Autodesk Inventor part; units mm, degrees
ref_plane "YZ Plane" through (0, 0, 0) normal (1, 0, 0) x (0, 1, 0)
ref_plane "XZ Plane" through (0, 0, 0) normal (0, 1, 0) x (-1, 0, 0)
ref_plane "XY Plane" through (0, 0, 0) normal (0, 0, 1) x (1, 0, 0)
sketch "Sketch1" plane through (0, 0, 0) normal (0, 0, 1) x (1, 0, 0)
  line L0 (18.1, 0) -> (18.1, 27)
  line L1 (18.1, 27) -> (-0.25, 27)
  line L2 (0, 0) -> (18.1, 0)
  circle A0 centre (13.6, 6.8375) radius 2.5
  circle A1 centre (13.6, 20.1625) radius 2.5
  line L3 (-104.55, 27) -> (-122.9, 27)
  line L4 (-122.9, 0) -> (-122.9, 27)
  line L5 (-104.55, 0) -> (-122.9, 0)
  circle A2 centre (-118.4, 6.8375) radius 2.5
  circle A3 centre (-118.4, 20.1625) radius 2.5
  line L6 (-104.55, 27) -> (-0.25, 27)
  line L7 (-104.55, 0) -> (0, 0)
extrude "Extrusion1" add sketch "Sketch1" along normal blind 10
hole "Hole1" at (13.6, 20.1625, 10) direction (0, 0, -1) diameter 8 depth 2
hole "Hole2" at (13.6, 6.8375, 10) direction (0, 0, -1) diameter 8 depth 2
hole "Hole3" at (-118.4, 20.1625, 10) direction (0, 0, -1) diameter 8 depth 2
hole "Hole4" at (-118.4, 6.8375, 10) direction (0, 0, -1) diameter 8 depth 2
chamfer "Chamfer1" [suppressed]
sketch "Sketch2" plane through (0, 0, 0) normal (0, 1, 0) x (-1, 0, 0)
  line L0 (-18.1, 0) -> (104.6, 0) construction
  circle A0 centre (6.05, 0) radius 5.75
  circle A1 centre (29.25, 0) radius 5.75
  circle A2 centre (52.45, 0) radius 5.75
  circle A3 centre (29.25, 0) radius 5.75
  circle A4 centre (75.65, 0) radius 5.75
  circle A5 centre (98.85, 0) radius 5.75
  line L1 (-18.1, 0) -> (0, 0) construction
  line L2 (122.9, 0) -> (122.9, 10)
  line L3 (122.9, 0) -> (122.9, 10)
  line L4 (-18.1, 0) -> (-18.1, 10)
  line L5 (-18.1, 0) -> (-18.1, 10)
  dimension "d49" = 11.5
  dimension "d50" = 23.2
  dimension "d51" = 23.2
  dimension "d52" = 23.2
  dimension "d54" = 23.2
  dimension "d55" = 23.2
extrude "Extrusion2" cut sketch "Sketch2" along normal through all
sketch "Sketch3" plane through (0, 0, 0) normal (0, 0, 1) x (1, 0, 0)
  line L0 (-69.9, 0) -> (-69.9, 27)
  line L1 (-58.2, 27) -> (-69.9, 27)
  line L2 (-58.2, 27) -> (-58.2, 0)
  line L3 (-69.9, 0) -> (-58.2, 0)
  line L4 (-35, 27) -> (-35, 0)
  line L5 (-46.7, 0) -> (-35, 0)
  line L6 (-46.7, 0) -> (-46.7, 27)
  line L7 (-35, 27) -> (-46.7, 27)
  circle A0 centre (-64.05, 13.5) radius 2.6
  circle A1 centre (-40.85, 13.5) radius 2.6
  line L8 (-69.9, 0) -> (-69.9, 27)
  line L9 (-69.9, 13.5) -> (-35, 13.5) construction
  line L10 (-64.05, 0) -> (-64.05, 27) construction
  line L11 (-122.9, 0) -> (18.1, 0)
  line L12 (-40.85, 0) -> (-40.85, 27) construction
  point P0 (0, 0)
  point P1 (-40.85, 13.5)
  dimension "d66" = 5.2
extrude "Extrusion3" cut sketch "Sketch3" along normal through all contours A0 | A1
hole "Hole5" at (-40.85, 13.5, 10) direction (0, 0, -1) diameter 9.5 depth 3
hole "Hole6" at (-64.05, 13.5, 10) direction (0, 0, -1) diameter 9.5 depth 3
equation "\"d51\" = d50"
equation "\"d52\" = d50"
equation "\"d54\" = d50"
properties part number "cylinder-holder-1" material "Nylon 6/6"
The model under review builds one solid part; all positions refer to its coordinate system, in mm. A direction names the side the tool comes from. Round coordinates to 2 decimals unless told otherwise and drop trailing zeros. Order: outer loops, then holes, each group sorted by start corner. A loop starts at its lowest first (then second) coordinate and runs counter-clockwise, first axis right, second up. Notation, with made-up numbers: (-28, 5.25) - (-5, 5.25) arc R20 ccw to (-5, 10.25) - close; hole circle Ø5 at (-34, 12). An arc over 180 degrees is marked (long way). Use one line per item in the form item = value.
Q1. Add section B-B on y = 13.5. Give the number of separate pieces and of enclosed holes in the cut face, then the cut area to 3 significant figures.
Response values:
separate_pieces = 3
enclosed_holes = 0
area = 1,020 mm^2
Q2. Clearance check with flat-ended pins moving along their axes: P1, Ø7.5, axis at x = -40.85, y = 13.5, coming from the +Z side; P2, Ø6, axis at x = 13.6, y = 20.16, coming from the +Z side. State where each tip first meets the part, or that it passes through.
Response values:
P1 = 7
P2 = 8
Q3. Add section D-D on x = -118.4. Give the boundary of the cut face in (y, z), then the cut area to 3 significant figures.
Response values:
outline = (0, 0) - (4.34, 0) - (4.34, 8) - (2.84, 8) - (2.84, 10) - (0, 10) - close; (9.34, 0) - (17.66, 0) - (17.66, 8) - (16.16, 8) - (16.16, 10) - (10.84, 10) - (10.84, 8) - (9.34, 8) - close; (22.66, 0) - (27, 0) - (27, 10) - (24.16, 10) - (24.16, 8) - (22.66, 8) - close
area = 158 mm^2
Q4. Tool access review of faces 1 (the flat face through (14, 4, 8)), 2 (the cylindrical face through (-120.384, 8.359, 3.944)): name each direction out of +Z, -Z, +X, -X, +Y, -Y from which nothing blocks a thin tool from reaching the whole face with its end or side.
Response values:
face_1 = +Z
face_2 = +Z, -Z
Q5. Add section A-A on x = -64.05. Give the boundary of the cut face in (y, z), then the cut area to 3 significant figures.
Response values:
outline = (0, 0) - (10.9, 0) - (10.9, 7) - (8.75, 7) - (8.75, 10) - (0, 10) - close; (16.1, 0) - (27, 0) - (27, 10) - (18.25, 10) - (18.25, 7) - (16.1, 7) - close
area = 205 mm^2
Q6. To check wall thickness, follow line 1 (Y direction, x = 13.6, z = 3); line 2 (X direction, y = 5, z = 6.75); line 3 (Y direction, x = -118.4, z = 9.55). State the ranges of each line that lie inside material, in increasing order.
Response values:
line_1 = 0 to 4.34, 9.34 to 17.66, 22.66 to 27
line_2 = -122.9 to -120.1, -116.7 to 11.9, 15.3 to 18.1
line_3 = 0 to 2.84, 10.84 to 16.16, 24.16 to 27
Q7. Mouldability with a two-part tool opening along X and no side actions: class faces 3 (the flat face through (12, 18, 8)), 4 (the flat face through (18.1, 13, 5)), 5 (the flat face through (-53, 14, 10)), 6 (the flat face through (-39, 11, 7)) as pulls with the +X half, pulls with the -X half, needs draft (parallel to the pull), parting line crosses it, or undercut.
Response values:
face_3 = undercut
face_4 = pulls with the +X half
face_5 = needs draft
face_6 = undercut
